from build123d import *

# Parameters (mm, degrees)
SKETCH1_R           = 1.5
BOSS_EXTRUDE1_DEPTH = 6
FILLET1_R           = 20
CUT_EXTRUDE1_REACH  = 125.376
SKETCH5_R           = 1.25
BOSS_EXTRUDE2_DEPTH = 6
FILLET2_R           = 3
SKETCH6_W           = 6
SKETCH6_H           = 30.707123962
SKETCH6_H_2         = 30.684410161
CUT_EXTRUDE2_DEPTH  = 1
FILLET3_R           = 1.5


with BuildPart() as part:
    # Sketch1 → Boss-Extrude1 (new body)
    with BuildSketch(Plane(origin=(0, 0, 0), x_dir=(1, 0, 0), z_dir=(0, 1, 0))):
        with BuildLine():
            Line((-63.952675545, 96.063842822), (0, 60))
            Line((0, 60), (63.952675545, 96.063842822))
            ThreePointArc((63.952675545, 96.063842822), (73.389179934, 94.898361774), (75.046634262, 85.5357336))
            Line((75.046634262, 85.5357336), (40, 15))
            Line((40, 15), (75.434864258, -86.457646081))
            ThreePointArc((75.434864258, -86.457646081), (72.068849374, -95.912520808), (62.113867032, -94.638535384))
            Line((62.113867032, -94.638535384), (0, -30))
            Line((0, -30), (-62.113867032, -94.638535384))
            ThreePointArc((-62.113867032, -94.638535384), (-72.068849374, -95.912520808), (-75.434864258, -86.457646081))
            Line((-75.434864258, -86.457646081), (-40, 15))
            Line((-40, 15), (-75.046634262, 85.5357336))
            ThreePointArc((-75.046634262, 85.5357336), (-73.389179934, 94.898361774), (-63.952675545, 96.063842822))
        make_face()
        with Locations(Location((-67.882250994, 89.09545443, 0), (0, 0, 270))):
            Circle(SKETCH1_R, mode=Mode.SUBTRACT)
        with Locations(Location((67.882250994, 89.09545443, 0), (0, 0, 270))):
            Circle(SKETCH1_R, mode=Mode.SUBTRACT)
        with Locations(Location((-67.882250994, -89.09545443, 0), (0, 0, 270))):
            Circle(SKETCH1_R, mode=Mode.SUBTRACT)
        with Locations(Location((67.882250994, -89.09545443, 0), (0, 0, 270))):
            Circle(SKETCH1_R, mode=Mode.SUBTRACT)
        with Locations(Location((-39, 65, 0), (0, 0, 270))):
            Circle(SKETCH1_R, mode=Mode.SUBTRACT)
        with Locations(Location((39, 65, 0), (0, 0, 270))):
            Circle(SKETCH1_R, mode=Mode.SUBTRACT)
        with Locations(Location((39, -55, 0), (0, 0, 270))):
            Circle(SKETCH1_R, mode=Mode.SUBTRACT)
        with Locations(Location((-39, -55, 0), (0, 0, 270))):
            Circle(SKETCH1_R, mode=Mode.SUBTRACT)
    extrude(amount=BOSS_EXTRUDE1_DEPTH)

    # Fillet1
    fillet1_edges = [part.edges().sort_by_distance(p)[0] for p in [
        (0, 3, -60),
        (40, 3, -15),
        (0, 3, 30),
        (-40, 3, -15),
    ]]
    fillet(fillet1_edges, radius=FILLET1_R)

    # Sketch2 → Cut-Extrude1 (cut, up to next)
    with BuildSketch(Plane(origin=(0, 6, 0), x_dir=(1, 0, 0), z_dir=(0, 1, 0)), mode=Mode.PRIVATE) as cut_extrude1_sk1:
        with BuildLine():
            Line((-44.444795008, 64.398316163), (-27.62775586, 30.551922116))
            ThreePointArc((-27.62775586, 30.551922116), (-23.732915732, 16.019014171), (-25.78366338, 1.113658522))
            Line((-25.78366338, 1.113658522), (-43.323179503, -49.105752685))
            Line((-43.323179503, -49.105752685), (-27.39982382, -32.535179334))
            ThreePointArc((-27.39982382, -32.535179334), (0, -20.864813867), (27.39982382, -32.535179334))
            Line((27.39982382, -32.535179334), (43.323179503, -49.105752685))
            Line((43.323179503, -49.105752685), (25.78366338, 1.113658522))
            ThreePointArc((25.78366338, 1.113658522), (23.732915732, 16.019014171), (27.62775586, 30.551922116))
            Line((27.62775586, 30.551922116), (44.444795008, 64.398316163))
            Line((44.444795008, 64.398316163), (18.665483383, 49.860987824))
            ThreePointArc((18.665483383, 49.860987824), (0, 44.96083269), (-18.665483383, 49.860987824))
            Line((-18.665483383, 49.860987824), (-44.444795008, 64.398316163))
        make_face()
    cut_extrude1_tool1 = extrude(cut_extrude1_sk1.sketch, amount=-CUT_EXTRUDE1_REACH, mode=Mode.PRIVATE) & part.part
    add(cut_extrude1_tool1.solids().sort_by_distance((0, 6, -11.306472))[0], mode=Mode.SUBTRACT)

    # Sketch5 → Boss-Extrude2 (add)
    with BuildSketch(Plane(origin=(0, 6, 0), x_dir=(1, 0, 0), z_dir=(0, 1, 0))):
        with BuildLine():
            Line((-26.321862123, 1.247557887), (0, -5.301102183))
            Line((0, -5.301102183), (26.321862123, 1.247557887))
            Line((26.321862123, 1.247557887), (27.770453283, -4.57494876))
            Line((27.770453283, -4.57494876), (4, -10.488839561))
            Line((4, -10.488839561), (4, -21.075926612))
            ThreePointArc((4, -21.075926612), (0, -20.864813867), (-4, -21.075926612))
            Line((-4, -21.075926612), (-4, -10.488839561))
            Line((-4, -10.488839561), (-27.770453283, -4.57494876))
            Line((-27.770453283, -4.57494876), (-26.321862123, 1.247557887))
        make_face()
        with Locations(Location((-10.3, -5.83, 0), (0, 0, 270))):
            Circle(SKETCH5_R, mode=Mode.SUBTRACT)
        with Locations(Location((10.3, -5.83, 0), (0, 0, 270))):
            Circle(SKETCH5_R, mode=Mode.SUBTRACT)
    extrude(amount=-BOSS_EXTRUDE2_DEPTH)

    # Fillet2
    fillet2_edges = [part.edges().sort_by_distance(p)[0] for p in [
        (-44.444795008, 3, -64.398316163),
        (44.444795008, 3, -64.398316163),
        (25.78366338, 3, -1.113658522),
        (43.323179503, 3, 49.105752685),
        (-43.323179503, 3, 49.105752685),
        (-25.78366338, 3, -1.113658522),
        (0, 3, 5.301102183),
        (-4, 3, 10.488839561),
        (-4, 3, 21.075926612),
        (4, 3, 21.075926612),
        (4, 3, 10.488839561),
        (27.770453283, 3, 4.57494876),
        (-27.770453283, 3, 4.57494876),
    ]]
    fillet(fillet2_edges, radius=FILLET2_R)

    # Sketch6 → Cut-Extrude2 (cut)
    with BuildSketch(Plane(origin=(0, 6, 0), x_dir=(1, 0, 0), z_dir=(0, 1, 0))):
        with Locations((-39, -58.353561981)):
            Rectangle(SKETCH6_W, SKETCH6_H)
        with Locations((39, -58.353561981)):
            Rectangle(SKETCH6_W, SKETCH6_H)
        with Locations((39, 68.342205081)):
            Rectangle(SKETCH6_W, SKETCH6_H_2)
        with Locations((-39, 68.342205081)):
            Rectangle(SKETCH6_W, SKETCH6_H_2)
    extrude(amount=-CUT_EXTRUDE2_DEPTH, mode=Mode.SUBTRACT)

    # Fillet3
    fillet3_edges = [part.edges().sort_by_distance(p)[0] for p in [
        (-36, 5.5, 43),
        (-42, 5.5, 43),
        (36, 5.5, 43),
        (42, 5.5, 43),
        (42, 5.5, -53),
        (-42, 5.5, -53),
    ]]
    fillet(fillet3_edges, radius=FILLET3_R)


solid = part.part
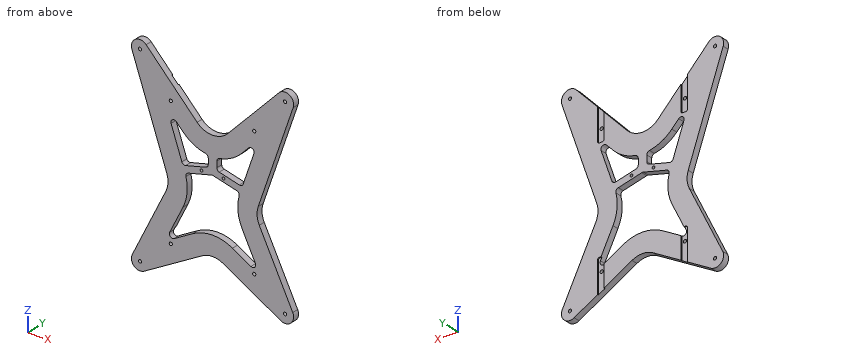
The listing builds one solid part. Answer for the finished solid, in the listing's coordinates (mm). Coordinates: 2 decimals unless noted, no trailing zeros. Write each loop counter-clockwise with the first axis right and the second up, starting at its lowest first coordinate (ties: lowest second). Pieces come first, ordered by that corner, then holes. Notation, with made-up numbers: (14, -10) - (67, -10) arc R34 cw to (67, 23) - close; hole circle Ø9 at (-8, -1). An arc over 180 degrees is marked (long way). Return JSON: item names as keys, results as strings.
1. Each of these flat-tipped pins is pushed along its axis until it touches: pin 1 Ø1.5 at (y, z) = (4.5, 9) entering from -X; pin 2 Ø1.5 at (y, z) = (1.5, 41.5) entering from -X (3 decimals); pin 3 Ø2 at (x, y) = (26, 4.5) entering from +Z; pin 4 Ø2.5 at (x, z) = (-67.88, 89.1) entering from +Y. Where does it stop, or does it pass through?
Final values:
{"pin 1": "x = -48.64", "pin 2": "x = -59.995", "pin 3": "z = 58.1", "pin 4": "through"}
2. The part is cut by section B-B on y = 2.15. Count the separate pieces of the cut face and the enclosed holes in it, then the cut area to 3 significant figures.
Final values:
{"separate pieces": "1", "enclosed holes": "13", "area": "12,200 mm^2"}
3. The part is cut by section C-C on z = -33. Determine the outline of the cut face in (x, y).
Final values:
{"outline": "(-48.94, 0) - (-28.84, 0) - (-28.84, 6) - (-48.94, 6) - close; (28.84, 0) - (48.94, 0) - (48.94, 6) - (28.84, 6) - close"}
4. The part is cut by section A-A on z = 71.5. Determine the outline of the cut face in (x, y).
Final values:
{"outline": "(-70.21, 0) - (-39.88, 0) - (-39.88, 5) - (-42, 5) - (-42, 6) - (-70.21, 6) - close; (39.88, 0) - (70.21, 0) - (70.21, 6) - (42, 6) - (42, 5) - (39.88, 5) - close"}
5. Consider line 1 along Z through (x, y) = (20, 3.05); line 2 along X through (y, z) = (2.55, -65); line 3 along Z through (x, y) = (-39, 2.15). Determine where each line is inside the solid, lowest interval first.
Final values:
{"line 1": "-71.28 to -50.61, 0.33 to 6.51, 26.55 to 50.81", "line 2": "-64.84 to -40.5, -37.5 to -8.8, 8.8 to 37.5, 40.5 to 64.84", "line 3": "-81.99 to -66.5, -63.5 to -59.54, -53.44 to 53.5, 56.5 to 70.59"}
